Input: part model. Units: mm. Frame: model coordinates. Face numbers are marked on the shaded views. Coordinates: 2 decimals unless noted, no trailing zeros. Write each loop counter-clockwise with the first axis right and the second up, starting at its lowest first coordinate (ties: lowest second). Pieces come first, ordered by that corner, then holes. Notation, with made-up numbers: (6, 68) - (52, 68) arc R20 ccw to (52, 99) - close; hole circle Ø4 at (24, 39.25). An arc over 180 degrees is marked (long way). Use a Markdown table: item, result. Add a question column.
Q1. Pin query (flat end, axial travel): P1, Ø12, axis at y = 17.5, z = -6.5, coming from the +X side; P2, Ø4, axis at x = -4.5, z = -7, coming from the -Y side; P3, Ø2, axis at x = 30.5, z = -4.5, coming from the -Y side. Return the tip coordinate at first contact, or that it passes through.
Q2. Section query A-A (y = 0). Return the cut outline in (x, z), then the cut area to 3 significant figures.
Q3. Section query B-B (x = -37.5). Return the cut outline in (y, z).
Q4. Mould query, pull axis Y, two halves, no side actions, for the marked faces 1, 2 and 3. Classes: released by +Y, released by -Y, zero draft, split by the parting line, or undercut.
Q5. Section query C-C (x = 31.25). Return the cut outline in (y, z).
Q6. Section query D-D (z = -7.5). Return the cut outline in (x, y), then the cut area to 3 significant figures.
Q7. Material intervals for probe 1 along Y at (x, z) = (-32.5, -14.25); probe 2 along Y at (x, z) = (33.5, -18.25); probe 3 along X at (y, z) = (54.5, -12), sorted ascending. Write a range as from..to.
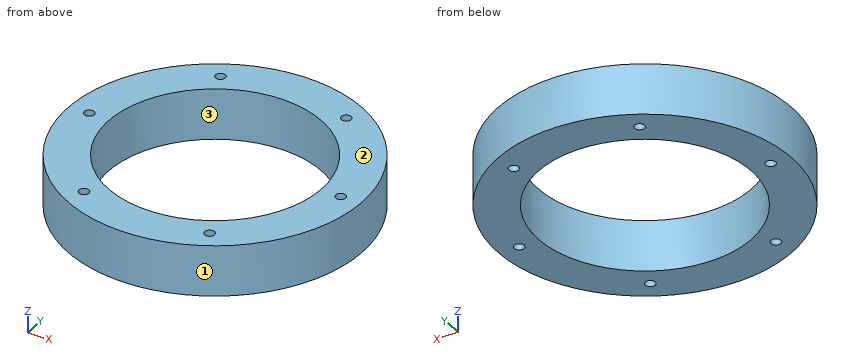
Autodesk Inventor part; units mm, degrees
ref_plane "Płaszczyzna konstrukcyjna1" through (0, 0, 0) normal (0, 0, 1) x (1, 0, 0)
ref_plane "YZ Plane" through (0, 0, 0) normal (1, 0, 0) x (0, 1, 0)
ref_plane "XZ Plane" through (0, 0, 0) normal (0, 1, 0) x (-1, 0, 0)
ref_plane "Płaszczyzna konstrukcyjna1" through (0, 0, 0) normal (0, 0, 1) x (1, 0, 0)
sketch "Szkic1" plane through (0, 0, 0) normal (0, 0, 1) x (1, 0, 0)
  circle A0 centre (0, 0) radius 72.5
  circle A1 centre (0, 0) radius 52.5
extrude "Wyciągnięcie proste1" add sketch "Szkic1" against normal blind 25
sketch "Szkic2" plane through (0, 0, -25) normal (0, 0, -1) x (-1, 0, 0)
  circle A0 centre (0, 0) radius 52.5
  line L0 (-52.5, 0) -> (-72.5, 0)
  circle A1 centre (0, 0) radius 72.5
  circle A2 centre (-62.5, 0) radius 3
  dimension "d2" = 20
  dimension "d3" = 6
hole "Otwór1" at (62.5, 0, -25) direction (0, 0, 1) diameter 4.917 end through all
pattern_circular "Szyk kołowy1" count 6 over 360 about axis through (0, 0, -10) along (0, 0, 1) of "Otwór1"
properties material "Stal nierdzewna"
Values follow:
| question | item | result |
|---|---|---|
| 1 | P1 | x = 71.58 |
| 1 | P2 | y = -72.46 |
| 1 | P3 | y = -66.23 |
| 2 | outline | (-72.5, -25) - (-64.96, -25) - (-64.96, 0) - (-72.5, 0) - close; (-60.04, -25) - (-52.5, -25) - (-52.5, 0) - (-60.04, 0) - close; (52.5, -25) - (60.04, -25) - (60.04, 0) - (52.5, 0) - close; (64.96, -25) - (72.5, -25) - (72.5, 0) - (64.96, 0) - close |
| 2 | area | 754 mm2 |
| 3 | outline | (-62.05, -25) - (-36.74, -25) - (-36.74, 0) - (-62.05, 0) - close; (36.74, -25) - (62.05, -25) - (62.05, 0) - (36.74, 0) - close |
| 4 | face 1 | split by the parting line |
| 4 | face 2 | zero draft |
| 4 | face 3 | undercut |
| 5 | outline | (-65.42, -25) - (-56.59, -25) - (-56.59, 0) - (-65.42, 0) - close; (-51.67, -25) - (-42.19, -25) - (-42.19, 0) - (-51.67, 0) - close; (42.19, -25) - (51.67, -25) - (51.67, 0) - (42.19, 0) - close; (56.59, -25) - (65.42, -25) - (65.42, 0) - (56.59, 0) - close |
| 6 | outline | circle Ø145 at (0, 0); hole circle Ø4.92 at (-62.5, 0); hole circle Ø105 at (0, 0); hole circle Ø4.92 at (-31.25, -54.13); hole circle Ø4.92 at (-31.25, 54.13); hole circle Ø4.92 at (31.25, -54.13); hole circle Ø4.92 at (31.25, 54.13); hole circle Ø4.92 at (62.5, 0) |
| 6 | area | 7,740 mm2 |
| 7 | probe 1 | -64.81..-56.24, -52.01..-41.23, 41.23..52.01, 56.24..64.81 |
| 7 | probe 2 | -64.3..-55.12, -53.14..-40.42, 40.42..53.14, 55.12..64.3 |
| 7 | probe 3 | -47.81..-33.68, -28.82..28.82, 33.68..47.81 |
